For this review, take the finished solid that the model builds, in its own axes (mm). A direction names the side the tool comes from. Coordinates: 2 decimals unless noted, no trailing zeros. Write each loop counter-clockwise with the first axis right and the second up, starting at its lowest first coordinate (ties: lowest second). Pieces come first, ordered by that corner, then holes. Notation, with made-up numbers: (80, 78) - (108, 78) arc R33 cw to (108, 114) - close; hole circle Ø10 at (-13.5, 83). An arc over 180 degrees is marked (long way). Write each question's results on one line, items separated by ' | '.
from build123d import *

# Parameters (mm, degrees)
F0_R     = 13
F0_R_2   = 1.5
F1_DEPTH = 6
F2_DEPTH = 6


# Not quite as in the source:
# - a feature names something its author has since deleted; it is built from what else it names


with BuildPart() as f1:
    # F0 (on Top) → F1 (new body)
    with BuildSketch(Plane.XY):
        Polygon((32, 18.4752086141), (16, 9.237604307), (16, -9.237604307), (32, -18.4752086141), (48, -9.237604307), (48, 9.237604307), align=None)
        with Locations((32, 0)):
            Circle(F0_R, mode=Mode.SUBTRACT)
        Polygon((16, -9.237604307), (16, 9.237604307), (0, 18.4752086141), (-2.5, 17.0318329411), (-5, 15.5884572681), (-16, 9.237604307), (-16, -9.237604307), (0, -18.4752086141), align=None)
        Circle(F0_R, mode=Mode.SUBTRACT)
        Polygon((0, 18.4752086141), (16, 9.237604307), (32, 18.4752086141), (32, 36.9504172281), (16, 46.1880215352), (0, 36.9504172281), (0, 22.805335633), (0, 21.36195996), align=None)
        with Locations((16, 27.7128129211)):
            Circle(F0_R, mode=Mode.SUBTRACT)
        Polygon((-2.5, 17.0318329411), (0, 18.4752086141), (0, 21.36195996), (-2.5, 22.805335633), (-5, 21.36195996), (-5, 18.4752086141), align=None)
        with Locations((-2.5, 19.918584287)):
            Circle(F0_R_2, mode=Mode.SUBTRACT)
        Polygon((32, 36.9504172281), (32, 18.4752086141), (48, 9.237604307), (64, 18.4752086141), (64, 36.9504172281), (48, 46.1880215352), align=None)
        with Locations((48, 27.7128129211)):
            Circle(F0_R, mode=Mode.SUBTRACT)
        Polygon((64, 18.4752086141), (48, 9.237604307), (48, -9.237604307), (64, -18.4752086141), (80, -9.237604307), (80, 9.237604307), align=None)
        with Locations((64, 0)):
            Circle(F0_R, mode=Mode.SUBTRACT)
        Polygon((16, 46.1880215352), (32, 36.9504172281), (48, 46.1880215352), (48, 64.6632301492), (32, 73.9008344563), (16, 64.6632301492), align=None)
        with Locations((32, 55.4256258422)):
            Circle(F0_R, mode=Mode.SUBTRACT)
        Polygon((64, 36.9504172281), (64, 18.4752086141), (80, 9.237604307), (96, 18.4752086141), (96, 36.9504172281), (80, 46.1880215352), align=None)
        with Locations((80, 27.7128129211)):
            Circle(F0_R, mode=Mode.SUBTRACT)
        Polygon((0, 36.9504172281), (16, 46.1880215352), (16, 64.6632301492), (0, 73.9008344563), (-2.5, 72.4574587833), (-5, 71.0140831103), (-16, 64.6632301492), (-16, 46.1880215352), align=None)
        with Locations((0, 55.4256258422)):
            Circle(F0_R, mode=Mode.SUBTRACT)
        Polygon((48, 64.6632301492), (48, 46.1880215352), (64, 36.9504172281), (80, 46.1880215352), (80, 64.6632301492), (64, 73.9008344563), align=None)
        with Locations((64, 55.4256258422)):
            Circle(F0_R, mode=Mode.SUBTRACT)
        Polygon((96, 18.4752086141), (80, 9.237604307), (80, -9.237604307), (96, -18.4752086141), (112, -9.237604307), (112, 9.237604307), align=None)
        with Locations((96, 0)):
            Circle(F0_R, mode=Mode.SUBTRACT)
        Polygon((32, 73.9008344563), (48, 64.6632301492), (64, 73.9008344563), (64, 92.3760430703), (48, 101.6136473774), (32, 92.3760430703), align=None)
        with Locations((48, 83.1384387633)):
            Circle(F0_R, mode=Mode.SUBTRACT)
        Polygon((96, 36.9504172281), (96, 18.4752086141), (112, 9.237604307), (128, 18.4752086141), (128, 36.9504172281), (112, 46.1880215352), align=None)
        with Locations((112, 27.7128129211)):
            Circle(F0_R, mode=Mode.SUBTRACT)
        Polygon((80, 64.6632301492), (80, 46.1880215352), (96, 36.9504172281), (112, 46.1880215352), (112, 64.6632301492), (96, 73.9008344563), align=None)
        with Locations((96, 55.4256258422)):
            Circle(F0_R, mode=Mode.SUBTRACT)
        Polygon((-2.5, 72.4574587833), (0, 73.9008344563), (0, 76.7875858022), (-2.5, 78.2309614752), (-5, 76.7875858022), (-5, 73.9008344563), align=None)
        with Locations((-2.5, 75.3442101292)):
            Circle(F0_R_2, mode=Mode.SUBTRACT)
        Polygon((64, 92.3760430703), (64, 73.9008344563), (80, 64.6632301492), (96, 73.9008344563), (96, 92.3760430703), (80, 101.6136473774), align=None)
        with Locations((80, 83.1384387633)):
            Circle(F0_R, mode=Mode.SUBTRACT)
        Polygon((128, 18.4752086141), (112, 9.237604307), (112, -9.237604307), (128, -18.4752086141), (144, -9.237604307), (144, 9.237604307), align=None)
        with Locations((128, 0)):
            Circle(F0_R, mode=Mode.SUBTRACT)
        Polygon((128, 36.9504172281), (128, 18.4752086141), (144, 9.237604307), (160, 18.4752086141), (160, 36.9504172281), (144, 46.1880215352), align=None)
        with Locations((144, 27.7128129211)):
            Circle(F0_R, mode=Mode.SUBTRACT)
        Polygon((112, 64.6632301492), (112, 46.1880215352), (128, 36.9504172281), (144, 46.1880215352), (144, 64.6632301492), (128, 73.9008344563), align=None)
        with Locations((128, 55.4256258422)):
            Circle(F0_R, mode=Mode.SUBTRACT)
        Polygon((96, 92.3760430703), (96, 73.9008344563), (112, 64.6632301492), (128, 73.9008344563), (128, 92.3760430703), (112, 101.6136473774), align=None)
        with Locations((112, 83.1384387633)):
            Circle(F0_R, mode=Mode.SUBTRACT)
        Polygon((160, 18.4752086141), (144, 9.237604307), (144, -9.237604307), (160, -18.4752086141), (176, -9.237604307), (176, 4.9074772881), (176, 6.3508529611), (176, 9.237604307), align=None)
        with Locations((160, 0)):
            Circle(F0_R, mode=Mode.SUBTRACT)
        Polygon((160, 36.9504172281), (160, 18.4752086141), (176, 9.237604307), (178.5, 10.68097998), (181, 12.124355653), (192, 18.4752086141), (192, 36.9504172281), (176, 46.1880215352), align=None)
        with Locations((176, 27.7128129211)):
            Circle(F0_R, mode=Mode.SUBTRACT)
        Polygon((144, 64.6632301492), (144, 46.1880215352), (160, 36.9504172281), (176, 46.1880215352), (176, 60.3331031303), (176, 61.7764788033), (176, 64.6632301492), (160, 73.9008344563), align=None)
        with Locations((160, 55.4256258422)):
            Circle(F0_R, mode=Mode.SUBTRACT)
        Polygon((128, 92.3760430703), (128, 73.9008344563), (144, 64.6632301492), (160, 73.9008344563), (160, 92.3760430703), (144, 101.6136473774), align=None)
        with Locations((144, 83.1384387633)):
            Circle(F0_R, mode=Mode.SUBTRACT)
        Polygon((160, 92.3760430703), (160, 73.9008344563), (176, 64.6632301492), (178.5, 66.1066058222), (181, 67.5499814952), (192, 73.9008344563), (192, 92.3760430703), (176, 101.6136473774), align=None)
        with Locations((176, 83.1384387633)):
            Circle(F0_R, mode=Mode.SUBTRACT)
    extrude(amount=F1_DEPTH)

    # F0 (on Top) → F2 (join)
    with BuildSketch(Plane.XY):
        Polygon((0, 18.4752086141), (16, 9.237604307), (32, 18.4752086141), (32, 36.9504172281), (16, 46.1880215352), (0, 36.9504172281), (0, 22.805335633), (0, 21.36195996), align=None)
        with Locations((16, 27.7128129211)):
            Circle(F0_R, mode=Mode.SUBTRACT)
        Polygon((0, 73.9008344563), (16, 64.6632301492), (32, 73.9008344563), (32, 92.3760430703), (16, 101.6136473774), (0, 92.3760430703), (0, 78.2309614752), (0, 76.7875858022), align=None)
        with Locations((16, 83.1384387633)):
            Circle(F0_R, mode=Mode.SUBTRACT)
        Polygon((178.5, 10.68097998), (176, 9.237604307), (176, 6.3508529611), (178.5, 4.9074772881), (181, 6.3508529611), (181, 9.237604307), align=None)
        with Locations((178.5, 7.7942286341)):
            Circle(F0_R_2, mode=Mode.SUBTRACT)
        Polygon((178.5, 66.1066058222), (176, 64.6632301492), (176, 61.7764788033), (178.5, 60.3331031303), (181, 61.7764788033), (181, 64.6632301492), align=None)
        with Locations((178.5, 63.2198544763)):
            Circle(F0_R_2, mode=Mode.SUBTRACT)
        Polygon((-5, 71.0140831103), (-2.5, 72.4574587833), (-5, 73.9008344563), align=None)
        Polygon((-2.5, 78.2309614752), (0, 76.7875858022), (0, 78.2309614752), align=None)
        Polygon((-2.5, 22.805335633), (0, 21.36195996), (0, 22.805335633), align=None)
        Polygon((-5, 15.5884572681), (-2.5, 17.0318329411), (-5, 18.4752086141), align=None)
        Polygon((176, 61.7764788033), (176, 60.3331031303), (178.5, 60.3331031303), align=None)
        Polygon((181, 67.5499814952), (178.5, 66.1066058222), (181, 64.6632301492), align=None)
        Polygon((178.5, 4.9074772881), (176, 6.3508529611), (176, 4.9074772881), align=None)
        Polygon((181, 12.124355653), (178.5, 10.68097998), (181, 9.237604307), align=None)
    extrude(amount=F2_DEPTH)


solid = f1.part
Q1. Take a section at A-A on y = -5. State the section outline as (x, z) points.
Results found:
outline: (-16, 0) - (-12, 0) - (-12, 6) - (-16, 6) - close; (12, 0) - (20, 0) - (20, 6) - (12, 6) - close; (44, 0) - (52, 0) - (52, 6) - (44, 6) - close; (76, 0) - (84, 0) - (84, 6) - (76, 6) - close; (108, 0) - (116, 0) - (116, 6) - (108, 6) - close; (140, 0) - (148, 0) - (148, 6) - (140, 6) - close; (172, 0) - (176, 0) - (176, 6) - (172, 6) - close
Q2. For faces 1 (the face through (119.9, -13.8, 3)), 2 (the face through (181, 9, 3)), 3 (the face through (-16, 56, 3)), 4 (the face through (184.112, 41.505, 2.958)), 5 (the face through (88.11, 96.93, 2.96)), list the 3-axis set-ups (+Z, -Z, +X, -X, +Y, -Y) from which the entire face can be reached by the end or side of a thin tool; tool diameter is ignored.
Results found:
face 1: +Z, -Z, -Y | face 2: +Z, -Z, +X, -Y | face 3: +Z, -Z, -X, +Y, -Y | face 4: +Z, -Z, +X | face 5: +Z, -Z, +Y
Q3. Take a section at C-C on y = 87. State the section outline as (x, z) points, plus the area to 3 significant figures.
Results found:
outline: (0, 0) - (3.59, 0) - (3.59, 6) - (0, 6) - close; (28.41, 0) - (35.59, 0) - (35.59, 6) - (28.41, 6) - close; (60.41, 0) - (67.59, 0) - (67.59, 6) - (60.41, 6) - close; (92.41, 0) - (99.59, 0) - (99.59, 6) - (92.41, 6) - close; (124.41, 0) - (131.59, 0) - (131.59, 6) - (124.41, 6) - close; (156.41, 0) - (163.59, 0) - (163.59, 6) - (156.41, 6) - close; (188.41, 0) - (192, 0) - (192, 6) - (188.41, 6) - close | area: 258 mm2
Q4. For pin 1 (1.8 mm diameter, centred on x = 178.5, y = 7.79, fed in from -Z); pin 2 (4 mm diameter, centred on x = -2.5, y = 75.34, fed in from +Z); pin 3 (3 mm diameter, centred on y = 65.5, z = 4, fed in from +X), all flat-tipped, find the tip position at first contact; note any pin that passes through.
Results found:
pin 1: through | pin 2: z = 6 | pin 3: x = 181
Q5. Take a section at B-B on x = 37.5. State the section outline as (y, z) points.
Results found:
outline: (-15.3, 0) - (-11.78, 0) - (-11.78, 6) - (-15.3, 6) - close; (11.78, 0) - (20.05, 0) - (20.05, 6) - (11.78, 6) - close; (35.38, 0) - (43.65, 0) - (43.65, 6) - (35.38, 6) - close; (67.2, 0) - (75.47, 0) - (75.47, 6) - (67.2, 6) - close; (90.8, 0) - (95.55, 0) - (95.55, 6) - (90.8, 6) - close
Q6. Wall thickness on line 1 along Y through (x, z) = (144, 2.55); line 2 along Y through (x, z) = (32, 4.4); line 3 along Y through (x, z) = (149, 0.5): over which ranges is each line inside the solid? List them lowest first. Write a range as from..to.
Results found:
line 1: -9.24..14.71, 40.71..70.14, 96.14..101.61 | line 2: -18.48..-13, 13..42.43, 68.43..92.38 | line 3: -12.12..-6.93, 6.93..15.71, 39.71..48.5, 62.35..71.14, 95.14..98.73
Q7. Take a section at D-D on x = 86. State the section outline as (y, z) points.
Results found:
outline: (-12.7, 0) - (-8.31, 0) - (-8.31, 6) - (-12.7, 6) - close; (8.31, 0) - (16.18, 0) - (16.18, 6) - (8.31, 6) - close; (39.25, 0) - (47.12, 0) - (47.12, 6) - (39.25, 6) - close; (63.73, 0) - (71.61, 0) - (71.61, 6) - (63.73, 6) - close; (94.67, 0) - (98.15, 0) - (98.15, 6) - (94.67, 6) - close
Q8. Mouldability with a two-part tool opening along Y and no side actions: class faces 6 (the face through (167.89, -13.92, 2.96)), 7 (the face through (56.11, 96.93, 2.96)), 8 (the face through (118.99, 94.1, 2.96)) as pulls with the +Y half, pulls with the -Y half, needs draft (parallel to the pull), parting line crosses it, or undercut.
Results found:
face 6: pulls with the -Y half | face 7: pulls with the +Y half | face 8: undercut
